Verification items for the finished model (mm, model axes). A direction names the side the tool comes from. Give positions to 0.01 mm unless a question says otherwise; leave off trailing zeros. Loops run counter-clockwise (first coordinate to the right, second up) from the corner with the lowest first, then second, coordinate; pieces in that order, holes last. Notation, with made-up numbers: (62.5, 17.25) -> (115.5, 17.25) arc R16 ccw to (115.5, 47.25) -> close; hole circle Ø5 at (42, 47). An arc over 180 degrees is marked (long way). Answer in a Markdown table with one row per item. Add a question column.
Q1. Material ranges on probe 1 along X at (y, z) = (1.1, -11.75); probe 2 along X at (y, z) = (4.45, 1.5); probe 3 along Z at (x, y) = (119, 5.25), recorded low to high.
Q2. Section check C-C on x = 119.5. Enter the section's corners in (y, z).
Q3. Release check for a two-part mould opening along X. For faces 5 (the face through (125, 3, 2)), 6 (the face through (86, 3, -14)), 7 (the face through (50.9, 3, -10)) record: pulls with the +X half, pulls with the -X half, needs draft (parallel to the pull), parting line crosses it, or undercut.
Q4. Set-up check for faces 1 (the face through (69, 0, -4)), 2 (the face through (48.333, 3, 2)), 3 (the face through (15, 3, 2)), 4 (the face through (69, 3, -8)): record each of +Z, -Z, +X, -X, +Y, -Y from which the full face is reachable in a straight line by a thin tool's end or side.
Q5. Section check B-B on x = 64.5. Enter the section's corners in (y, z), and give its area (3 significant figures).
Q6. Gauge pin test, flat ends, axial feed: P1, Ø1, axis at x = 63, y = 2, coming from the -Z side; P2, Ø1.5, axis at y = 4, z = -11.5, coming from the -X side; P3, Ø2, axis at y = 3.5, z = -7, coming from the +X side. Record the tip position at first contact, or that the pin passes through.
Q7. Section check A-A on z = -10.5. Enter the section's corners in (x, y), and give its area (3 significant figures).
```python
from build123d import *

# Parameters (mm, degrees)
SKETCH1_W               = 140
SKETCH1_H               = 8
BOSS_EXTRUDE1_DEPTH     = 6
SKETCH234_W             = 10
SKETCH234_H             = 6
BOSS_EXTRUDE234_DEPTH   = 6
FILLET134_R             = 1
SKETCH2341_W            = 10
SKETCH2341_H            = 6
BOSS_EXTRUDE2341_DEPTH  = 6
FILLET1341_R            = 1
SKETCH2342_W            = 10
SKETCH2342_H            = 6
BOSS_EXTRUDE2342_DEPTH  = 6
FILLET1342_R            = 1
SKETCH2343_W            = 10
SKETCH2343_H            = 6
BOSS_EXTRUDE2343_DEPTH  = 6
FILLET1343_R            = 1
SKETCH2344_W            = 10
SKETCH2344_H            = 6
BOSS_EXTRUDE2344_DEPTH  = 6
FILLET1344_R            = 1
SKETCH2346_W            = 10
SKETCH2346_H            = 6
BOSS_EXTRUDE2346_DEPTH  = 6
FILLET1346_R            = 1
FILLET1347_R            = 5
SKETCH23410_W           = 6
SKETCH23410_H           = 6
BOSS_EXTRUDE23410_DEPTH = 6
FILLET13411_R           = 1


with BuildPart() as part:
    # Sketch1 → Boss-Extrude1 (new body)
    with BuildSketch(Plane(origin=(0, 0, 0), x_dir=(1, 0, 0), z_dir=(0, 1, 0))):
        with Locations((70, 4)):
            Rectangle(SKETCH1_W, SKETCH1_H)
    extrude(amount=BOSS_EXTRUDE1_DEPTH)

    # Sketch234 → Boss-Extrude234 (add)
    with BuildSketch(Plane(origin=(119.232221392, 0, 0), x_dir=(1, 0, 0), z_dir=(0, 0, 1))):
        with Locations((0.767778608, 3)):
            Rectangle(SKETCH234_W, SKETCH234_H)
    extrude(amount=BOSS_EXTRUDE234_DEPTH)

    # Fillet134
    fillet134_edges = [part.edges().sort_by_distance(p)[0] for p in [
        (115, 3, 6),
        (125, 3, 6),
    ]]
    fillet(fillet134_edges, radius=FILLET134_R)

    # Sketch2341 → Boss-Extrude2341 (add)
    with BuildSketch(Plane(origin=(85.898888059, 0, 0), x_dir=(1, 0, 0), z_dir=(0, 0, 1))):
        with Locations((0.767778608, 3)):
            Rectangle(SKETCH2341_W, SKETCH2341_H)
    extrude(amount=BOSS_EXTRUDE2341_DEPTH)

    # Fillet1341
    fillet1341_edges = [part.edges().sort_by_distance(p)[0] for p in [
        (91.666666667, 3, 6),
        (81.666666667, 3, 6),
    ]]
    fillet(fillet1341_edges, radius=FILLET1341_R)

    # Sketch2342 → Boss-Extrude2342 (add)
    with BuildSketch(Plane(origin=(52.565554726, 0, 0), x_dir=(1, 0, 0), z_dir=(0, 0, 1))):
        with Locations((0.767778608, 3)):
            Rectangle(SKETCH2342_W, SKETCH2342_H)
    extrude(amount=BOSS_EXTRUDE2342_DEPTH)

    # Fillet1342
    fillet1342_edges = [part.edges().sort_by_distance(p)[0] for p in [
        (58.333333333, 3, 6),
        (48.333333333, 3, 6),
    ]]
    fillet(fillet1342_edges, radius=FILLET1342_R)

    # Sketch2343 → Boss-Extrude2343 (add)
    with BuildSketch(Plane(origin=(19.232221392, 0, 0), x_dir=(1, 0, 0), z_dir=(0, 0, 1))):
        with Locations((0.767778608, 3)):
            Rectangle(SKETCH2343_W, SKETCH2343_H)
    extrude(amount=BOSS_EXTRUDE2343_DEPTH)

    # Fillet1343
    fillet1343_edges = [part.edges().sort_by_distance(p)[0] for p in [
        (25, 3, 6),
        (15, 3, 6),
    ]]
    fillet(fillet1343_edges, radius=FILLET1343_R)

    # Sketch2344 → Boss-Extrude2344 (add)
    with BuildSketch(Plane(origin=(84.932221392, 6, -8), x_dir=(1, 0, 0), z_dir=(0, 0, -1))):
        with Locations((0.767778608, 3)):
            Rectangle(SKETCH2344_W, SKETCH2344_H)
    extrude(amount=BOSS_EXTRUDE2344_DEPTH)

    # Fillet1344
    fillet1344_edges = [part.edges().sort_by_distance(p)[0] for p in [
        (80.7, 3, -14),
        (90.7, 3, -14),
    ]]
    fillet(fillet1344_edges, radius=FILLET1344_R)

    # Sketch2346 → Boss-Extrude2346 (add)
    with BuildSketch(Plane(origin=(11.432221392, 6, -8), x_dir=(1, 0, 0), z_dir=(0, 0, -1))):
        with Locations((0.767778608, 3)):
            Rectangle(SKETCH2346_W, SKETCH2346_H)
    extrude(amount=BOSS_EXTRUDE2346_DEPTH)

    # Fillet1346
    fillet1346_edges = [part.edges().sort_by_distance(p)[0] for p in [
        (17.2, 3, -14),
        (7.2, 3, -14),
    ]]
    fillet(fillet1346_edges, radius=FILLET1346_R)

    # Fillet1347
    fillet1347_edges = [part.edges().sort_by_distance(p)[0] for p in [
        (140, 3, -8),
    ]]
    fillet(fillet1347_edges, radius=FILLET1347_R)

    # Sketch23410 → Boss-Extrude23410 (add)
    with BuildSketch(Plane(origin=(53.132221392, 6, -8), x_dir=(1, 0, 0), z_dir=(0, 0, -1))):
        with Locations((0.767778608, 3)):
            Rectangle(SKETCH23410_W, SKETCH23410_H)
    extrude(amount=BOSS_EXTRUDE23410_DEPTH)

    # Fillet13411
    fillet13411_edges = [part.edges().sort_by_distance(p)[0] for p in [
        (56.9, 3, -14),
        (50.9, 3, -14),
    ]]
    fillet(fillet13411_edges, radius=FILLET13411_R)


solid = part.part
```
Taken from the geometry:
| question | item | result |
|---|---|---|
| 1 | probe 1 | x = 7.2 to 17.2, 50.9 to 56.9, 80.7 to 90.7 |
| 1 | probe 2 | x = 15 to 25, 48.33 to 58.33, 81.67 to 91.67, 115 to 125 |
| 1 | probe 3 | z = -8 to 6 |
| 2 | outline | (0, -8) -> (6, -8) -> (6, 6) -> (0, 6) -> close |
| 3 | face 5 | pulls with the +X half |
| 3 | face 6 | needs draft |
| 3 | face 7 | undercut |
| 4 | face 1 | +Z, -Z, +X, -X, -Y |
| 4 | face 2 | +Z, +Y, -Y |
| 4 | face 3 | +Z, -X, +Y, -Y |
| 4 | face 4 | -Z, +Y, -Y |
| 5 | outline | (0, -8) -> (6, -8) -> (6, 0) -> (0, 0) -> close |
| 5 | area | 48.0 mm² |
| 6 | P1 | stops at z = -8 |
| 6 | P2 | stops at x = 7.2 |
| 6 | P3 | stops at x = 139 |
| 7 | outline | (7.2, 0) -> (17.2, 0) -> (17.2, 6) -> (7.2, 6) -> close; (50.9, 0) -> (56.9, 0) -> (56.9, 6) -> (50.9, 6) -> close; (80.7, 0) -> (90.7, 0) -> (90.7, 6) -> (80.7, 6) -> close |
| 7 | area | 156 mm² |
